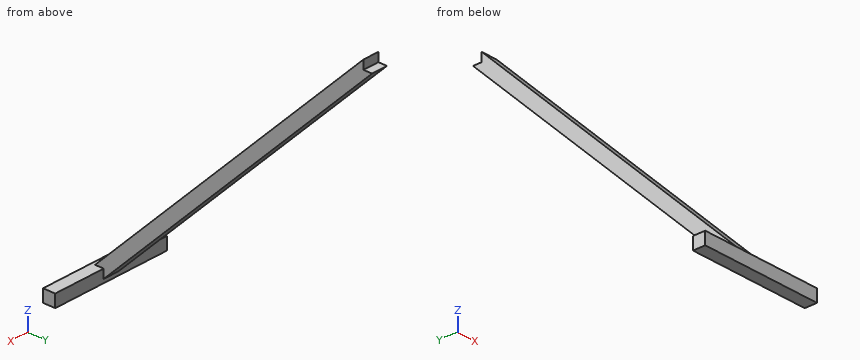
```python
from build123d import *

# Parameters (mm, degrees)
F1_DEPTH = 10
F2_DEPTH = 75


with BuildPart() as f1:
    # F0 (on Right) → F1 (new body, symmetric)
    with BuildSketch(Plane.YZ):
        Polygon((149.497071, 227.858104), (-179.307582, -100.946549), (-168.700981, -100.946549), (-168.700981, -111.553151), (160.103673, 217.251502), (149.497071, 217.251502), align=None)
    extrude(amount=F1_DEPTH, both=True)

    # F0 (on Right) → F2 (join, symmetric)
    with BuildSketch(Plane.YZ):
        Polygon((-168.700981, -111.553151), (-179.307582, -100.946549), (-183.700981, -100.946549), (-183.700981, -115.946549), (-168.700981, -115.946549), align=None)
        Polygon((-168.700981, -100.946549), (-179.307582, -100.946549), (-168.700981, -111.553151), align=None)
    extrude(amount=F2_DEPTH, both=True)


solid = f1.part
```
CAD build for the part. Positions are in the model's coordinates, mm. Coordinates: 2 decimals unless noted, no trailing zeros. Order: outer loops, then holes, each group sorted by start corner. A loop starts at its lowest first (then second) coordinate and runs counter-clockwise, first axis right, second up. Notation, with made-up numbers: (-15, 59.25) - (12, 59.25) arc R23 ccw to (12, 70.25) - close; hole circle Ø6 at (89, 60). An arc over 180 degrees is marked (long way). Use a Markdown table: item, result. Add a question column.
(1) Flat gauge pins, fed straight in: pin 1 (11.5 mm diameter, centred on x = 0, y = 154.5, fed in from +Z); pin 2 (4.5 mm diameter, centred on x = -36.5, z = -108.5, fed in from +Y); pin 3 (5.5 mm diameter, centred on x = -2, z = 224.5, fed in from +Y). Where does each tip first touch, or does it go through?
(2) Saw through at A-A (x = -47). Give the cut face in (y, z).
(3) Drill centre line: line 1 along X through (y, z) = (120, 185.5). Where is it in solid material? Low to high. Write a range as [from, to].
(4) Saw through at B-B (z = 83.5). Give the cut face in (x, y).
Solved:
| question | item | result |
|---|---|---|
| 1 | pin 1 | stops at z = 227.86 |
| 1 | pin 2 | stops at y = -168.7 |
| 1 | pin 3 | stops at y = 149.5 |
| 2 | outline | (-183.7, -115.95) - (-168.7, -115.95) - (-168.7, -100.95) - (-183.7, -100.95) - close |
| 3 | line 1 | x = [-10, 10] |
| 4 | outline | (-10, 5.14) - (10, 5.14) - (10, 26.35) - (-10, 26.35) - close |
